Drawing for the job (mm, zero at the part's lowest x, y, z). A direction names the side the tool comes from. Coordinates: 2 decimals unless noted, no trailing zeros. Loops run counter-clockwise (first coordinate to the right, second up) from the corner with the lowest first, then second, coordinate; pieces in that order, holes last. Notation, with made-up numbers: (29.5, 44) - (43.5, 44) arc R26 cw to (43.5, 76) - close; hole circle Ø6 at (61.5, 24.5). An arc over 180 degrees is marked (long way). Put each result on its own line as item: value.
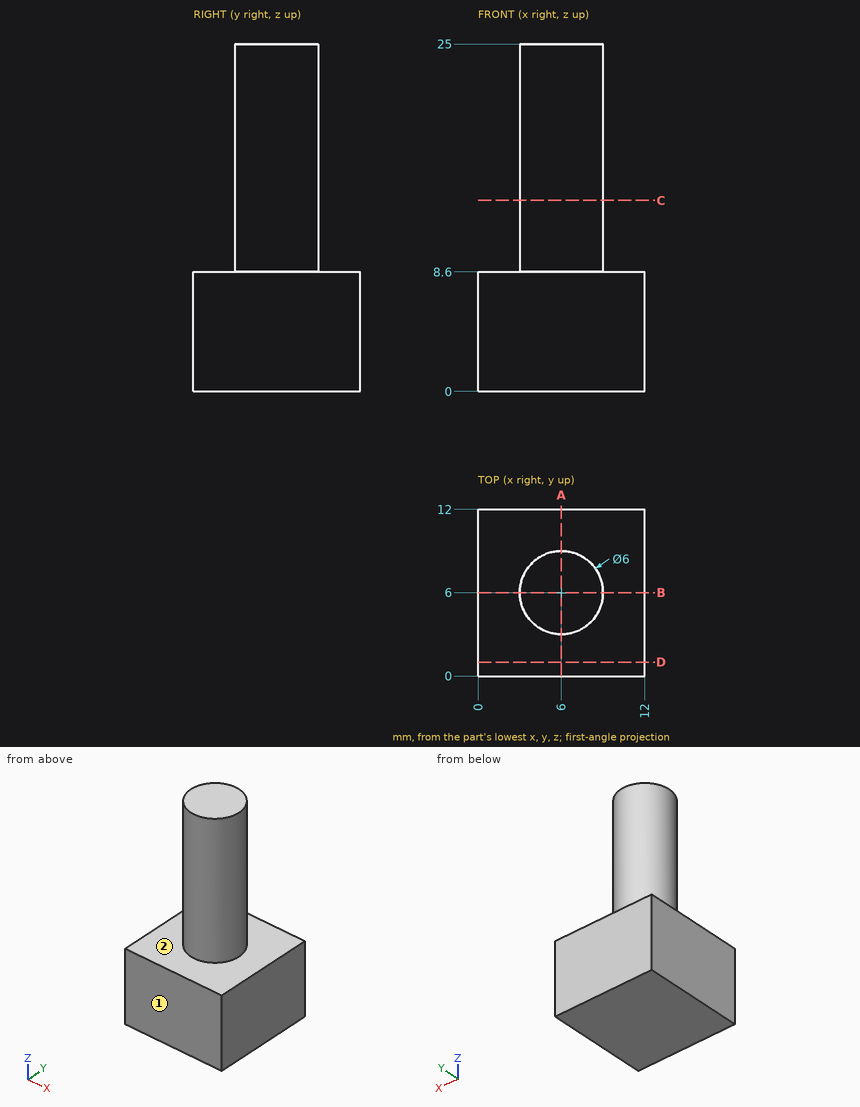
Q1. Tool access for the marked faces 1 and 2: list every direction of +Z, -Z, +X, -X, +Y, -Y with a clear straight run to the whole face (end or side of a thin tool).
Determined:
face 1: +Z, -Z, +X, -X, -Y
face 2: +Z
Q2. Pin check, flat tips, straight feed: pin 1 Ø2 at (x, z) = (8.5, 20.5) entering from -Y; pin 2 Ø2 at (y, z) = (6.5, 11.5) entering from +X; pin 3 Ø5 at (x, z) = (6.5, 15.5) entering from +Y. Stop position of each tip, or through.
Determined:
pin 1: y = 3.4
pin 2: x = 9
pin 3: y = 9
Q3. Slice it at C-C, the plane z = 13.75. Give the cut face in (x, y), then the cut area to 3 significant figures.
Determined:
outline: circle Ø6 at (6, 6)
area: 28.3 mm2
Q4. Slice it at D-D, the plane y = 1. Give the cut face in (x, z).
Determined:
outline: (0, 0) - (12, 0) - (12, 8.6) - (0, 8.6) - close
Q5. Slice it at A-A, the plane x = 6. Give the cut face in (y, z).
Determined:
outline: (0, 0) - (12, 0) - (12, 8.6) - (9, 8.6) - (9, 25) - (3, 25) - (3, 8.6) - (0, 8.6) - close
Q6. Wall check: L1, parallel to Z at x = 2, y = 6.5; L2, parallel to Y at x = 6, z = 13.25. Give the ranges that are in metal, low to high. Write a range as from..to.
Determined:
L1: 0..8.6
L2: 3..9
